Input: part model. Units: mm. Frame: model coordinates. A direction names the side the tool comes from. Round coordinates to 2 decimals unless told otherwise and drop trailing zeros. Loops run counter-clockwise (first coordinate to the right, second up) from the corner with the lowest first, then second, coordinate; pieces in that order, holes last. Notation, with made-up numbers: (80, -9.75) -> (139, -9.75) arc R20 ccw to (139, 3.25) -> close; hole circle Ø10 at (-35.5, 2). An arc over 180 degrees is marked (long way). Answer in a Markdown table with one row per item. Add a question column.
Q1. Section C-C, the plane z = 6.25. Output: boundary loops of the cut face in (x, y).
Q2. Pin query (flat end, axial travel): pin 1 (1.5 mm diameter, centred on x = 39.32, z = 3.85, fed in from +Y). Return the tip coordinate at first contact, or that it passes through.
Q3. Section A-A, the plane y = 0. Output: boundary loops of the cut face in (x, z), and give its area (3 significant figures).
Q4. Section D-D, the plane x = -10. Output: boundary loops of the cut face in (y, z).
Q5. Section B-B, the plane x = 25. Output: boundary loops of the cut face in (y, z).
Q6. Ray query, L1, parallel to Y at x = -10, z = 5.5; L2, parallel to Y at x = 38, z = 7.75; L3, parallel to X at y = -1.5, z = 7. Return the intervals inside material, ascending. Write a range as from..to.
Q7. Mould query, pull axis Z, two halves, no side actions, for faces 1 (the face through (-1, 0, 8)), 2 (the face through (40.246, 5.035, 4.69)), 3 (the face through (-42.747, 0.121, 3.944)). Classes: pulls with the +Z half, pulls with the -Z half, needs draft (parallel to the pull), parting line crosses it, or undercut.
Q8. Reachability of faces 4 (the face through (20.753, 0.149, 3.944)), 5 (the face through (37, 2.5, 4)) from +Z, -Z, +X, -X, +Y, -Y: full face, straight path, thin tool, end or side. Return the list, or none.
```python
from build123d import *

# Parameters (mm, degrees)
SKIZZE1_W                       = 100
SKIZZE1_H                       = 15
SKIZZE1_R                       = 2.75
SKIZZE1_R_2                     = 4.25
AUFSATZ_LINEAR_AUSTRAGEN1_DEPTH = 8
VERRUNDUNG1_R                   = 3
SCHNITT_LINEAR_AUSTRAGEN1_DEPTH = 30
M3_GEWINDEBOHRUNG1_D            = 2.5
VERRUNDUNG2_R                   = 5


with BuildPart() as part:
    # Skizze1 → Aufsatz-Linear austragen1 (new body)
    with BuildSketch(Plane.XY):
        Rectangle(SKIZZE1_W, SKIZZE1_H)
        with Locations((-10, 0)):
            Circle(SKIZZE1_R, mode=Mode.SUBTRACT)
        with Locations((-40, 0)):
            Circle(SKIZZE1_R, mode=Mode.SUBTRACT)
        with Locations((25, 0)):
            Circle(SKIZZE1_R_2, mode=Mode.SUBTRACT)
    extrude(amount=AUFSATZ_LINEAR_AUSTRAGEN1_DEPTH)

    # Verrundung1
    verrundung1_edges = [part.edges().sort_by_distance(p)[0] for p in [
        (-50, 7.5, 4),
        (50, 7.5, 4),
        (50, -7.5, 4),
        (-50, -7.5, 4),
    ]]
    fillet(verrundung1_edges, radius=VERRUNDUNG1_R)

    # Skizze2 → Schnitt-Linear austragen1 (cut)
    with BuildSketch(Plane.XY.offset(8)):
        with BuildLine():
            Line((25, 2.5), (52.731650319, 2.5))
            ThreePointArc((52.731650319, 2.5), (55.231650319, 0), (52.731650319, -2.5))
            Line((52.731650319, -2.5), (25, -2.5))
            ThreePointArc((25, -2.5), (22.5, 0), (25, 2.5))
        make_face()
    extrude(amount=-SCHNITT_LINEAR_AUSTRAGEN1_DEPTH, mode=Mode.SUBTRACT)

    # M3 Gewindebohrung1 (through all)
    with Locations(Plane.XZ.offset(7.5)):
        with Locations((39.324789102, 3.845615986)):
            Hole(M3_GEWINDEBOHRUNG1_D / 2)

    # Verrundung2
    # the kernel refuses this fillet: 5 mm, written as the material it takes off along each edge
    with BuildSketch(Plane(origin=(50, -2.5, 18), x_dir=(-1, 0, 0), z_dir=(0, 0, -1))) as verrundung2_piece_1:
        with BuildLine():
            CenterArc((4, -5), VERRUNDUNG2_R, 90, 53.130102354)
            Line((0, -2), (-0.08, -1.94))
            ThreePointArc((-0.08, -1.94), (-0.1, -1), (-0.1, 0))
            Line((-0.1, 0), (0, 0.1))
            Line((0, 0.1), (4, 0.1))
            Line((4, 0.1), (4, 0))
        make_face()
    extrude(amount=28, mode=Mode.SUBTRACT)
    with BuildSketch(Plane(origin=(50, 2.5, -10), x_dir=(0, 1, 0), z_dir=(0, 0, 1))) as verrundung2_piece_2:
        with BuildLine():
            CenterArc((5, 4), VERRUNDUNG2_R, 180, 53.130102354)
            Line((0, 4), (-0.1, 4))
            Line((-0.1, 4), (-0.1, 0))
            Line((-0.1, 0), (0, -0.1))
            ThreePointArc((0, -0.1), (1, -0.1), (1.94, -0.08))
            Line((1.94, -0.08), (2, 0))
        make_face()
    extrude(amount=28, mode=Mode.SUBTRACT)


solid = part.part
```
Answer block:
| question | item | result |
|---|---|---|
| 1 | outline | (-50, -4.5) arc R3 ccw to (-47, -7.5) -> (47, -7.5) arc R3 ccw to (50, -4.5) arc R5 ccw to (46, -2.5) -> (28.44, -2.5) arc R4.25 cw (long way) to (28.44, 2.5) -> (46, 2.5) arc R5 ccw to (50, 4.5) arc R3 ccw to (47, 7.5) -> (-47, 7.5) arc R3 ccw to (-50, 4.5) -> close; hole circle Ø5.5 at (-40, 0); hole circle Ø5.5 at (-10, 0) |
| 2 | pin 1 | through |
| 3 | outline | (-50, 0) -> (-42.75, 0) -> (-42.75, 8) -> (-50, 8) -> close; (-37.25, 0) -> (-12.75, 0) -> (-12.75, 8) -> (-37.25, 8) -> close; (-7.25, 0) -> (20.75, 0) -> (20.75, 8) -> (-7.25, 8) -> close |
| 3 | area | 478 mm^2 |
| 4 | outline | (-7.5, 0) -> (-2.75, 0) -> (-2.75, 8) -> (-7.5, 8) -> close; (2.75, 0) -> (7.5, 0) -> (7.5, 8) -> (2.75, 8) -> close |
| 5 | outline | (-7.5, 0) -> (-4.25, 0) -> (-4.25, 8) -> (-7.5, 8) -> close; (4.25, 0) -> (7.5, 0) -> (7.5, 8) -> (4.25, 8) -> close |
| 6 | L1 | -7.5..-2.75, 2.75..7.5 |
| 6 | L2 | -7.5..-2.5, 2.5..7.5 |
| 6 | L3 | -50..-42.3, -37.7..-12.3, -7.7..21.02 |
| 7 | face 1 | pulls with the +Z half |
| 7 | face 2 | undercut |
| 7 | face 3 | needs draft |
| 8 | face 4 | +Z, -Z |
| 8 | face 5 | +Z, -Z, +X |
